from build123d import *

# Parameters (mm, degrees)
SKETCH1_W           = 50
SKETCH1_H           = 50
BOSS_EXTRUDE1_DEPTH = 10
SKETCH2_W           = 5
SKETCH2_H           = 5
CUT_EXTRUDE1_DEPTH  = 6
SKETCH3_R           = 4
CUT_EXTRUDE2_DEPTH  = 0.5


with BuildPart() as part:
    # Sketch1 → Boss-Extrude1 (new body)
    with BuildSketch(Plane(origin=(0, 0, 0), x_dir=(1, 0, 0), z_dir=(0, 1, 0))):
        Rectangle(SKETCH1_W, SKETCH1_H)
    extrude(amount=BOSS_EXTRUDE1_DEPTH)

    # Sketch2 → Cut-Extrude1 (cut)
    with BuildSketch(Plane.ZY.offset(25)):
        with Locations((0, 5)):
            Rectangle(SKETCH2_W, SKETCH2_H)
    extrude(amount=-CUT_EXTRUDE1_DEPTH, mode=Mode.SUBTRACT)

    # Sketch3 → Cut-Extrude2 (cut)
    with BuildSketch(Plane(origin=(25, 0, 0), x_dir=(0, 0, -1), z_dir=(1, 0, 0))):
        with Locations((-12.5, 5)):
            Circle(SKETCH3_R)
        with Locations((12.5, 5)):
            Circle(SKETCH3_R)
        with Locations((0, 5)):
            Circle(SKETCH3_R)
    extrude(amount=-CUT_EXTRUDE2_DEPTH, mode=Mode.SUBTRACT)


solid = part.part
Geometry check sheet. Reference: the model listing, model coordinates, mm. A direction names the side the tool comes from. Give positions to 0.01 mm unless a question says otherwise; leave off trailing zeros. Write each loop counter-clockwise with the first axis right and the second up, starting at its lowest first coordinate (ties: lowest second). Pieces come first, ordered by that corner, then holes.
1) Cross-section at B-B (z = 0). Record the boundary of the cut face in (x, y), plus the area to 3 significant figures.
Values follow:
outline: (-25, 0) - (25, 0) - (25, 1) - (24.5, 1) - (24.5, 9) - (25, 9) - (25, 10) - (-25, 10) - (-25, 7.5) - (-19, 7.5) - (-19, 2.5) - (-25, 2.5) - close
area: 466 mm2
2) Cross-section at A-A (y = 5). Record the boundary of the cut face in (x, z).
Values follow:
outline: (-25, -25) - (25, -25) - (25, -16.5) - (24.5, -16.5) - (24.5, -8.5) - (25, -8.5) - (25, -4) - (24.5, -4) - (24.5, 4) - (25, 4) - (25, 8.5) - (24.5, 8.5) - (24.5, 16.5) - (25, 16.5) - (25, 25) - (-25, 25) - (-25, 2.5) - (-19, 2.5) - (-19, -2.5) - (-25, -2.5) - close
3) Thickness scan on line 1 (Y direction, x = 24.85, z = 12.5); line 2 (X direction, y = 2.5, z = 11); line 3 (X direction, y = 5.5, z = 2). Record the ranges inside material, lowest first.
Values follow:
line 1: y = 0 to 1, 9 to 10
line 2: x = -25 to 24.5
line 3: x = -19 to 24.5
4) Go/stop test with flat-tipped pins: pin 1 Ø2.5 at (y, z) = (4, 12.5) entering from +X; pin 2 Ø1 at (y, z) = (7.5, -15) entering from +X; pin 3 Ø1.5 at (y, z) = (4.5, -0.5) entering from -X. Record where each tip stops, or that it passes through.
Values follow:
pin 1: stops at x = 24.5
pin 2: stops at x = 25
pin 3: stops at x = -19
5) Set-up check for faces 1 (the face through (-19, 5, 0)), 2 (the face through (0, 5, -25)), 3 (the face through (24.5, 5, 0)): record each of +Z, -Z, +X, -X, +Y, -Y from which the full face is reachable in a straight line by a thin tool's end or side.
Values follow:
face 1: -X
face 2: -Z, +X, -X, +Y, -Y
face 3: +X
6) Release check for a two-part mould opening along Y. For faces 4 (the face through (25, 0.5, 0.3)), 5 (the face through (-22, 5, -2.5)), 6 (the face through (0, 10, 0)) record: released by +Y, released by -Y, zero draft, split by the parting line, or undercut.
Values follow:
face 4: zero draft
face 5: undercut
face 6: released by +Y
